Check sheet for the modelled part. Datum: model origin and axes. Units: mm. Face numbers are marked on the shaded views. Give positions to 0.01 mm unless a question says otherwise; leave off trailing zeros. Loops run counter-clockwise (first coordinate to the right, second up) from the corner with the lowest first, then second, coordinate; pieces in that order, holes last. Notation, with made-up numbers: M 18.25,-20.75 L 54.25,-20.75 A32 ccw 54.25,11.25 Z; hole C 72.25,-34.75 d3. An arc over 180 degrees is marked long. Use one line per item in the form item = value.
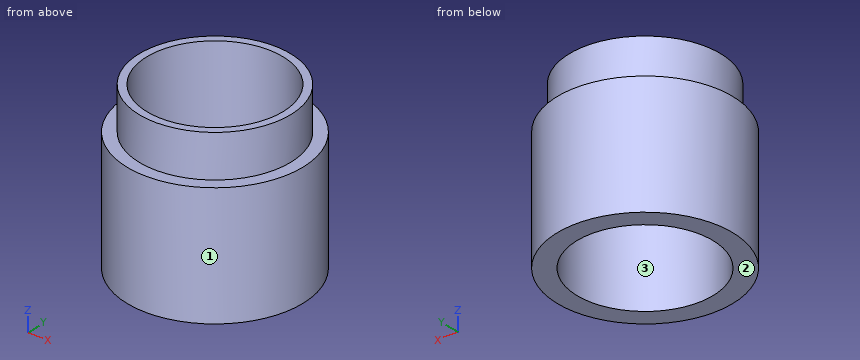
from build123d import *

# Parameters (mm, degrees)
SKETCH1_R           = 14.5
BOSS_EXTRUDE1_DEPTH = 13.5
SKETCH2_OUTSIDE_W   = 40.82
SKETCH2_OUTSIDE_H   = 40.82
SKETCH2_OUTSIDE_R   = 12.5
CUT_EXTRUDE1_DEPTH  = 7
SKETCH3_R           = 11.25
CUT_EXTRUDE2_DEPTH  = 34.904277016


with BuildPart() as part:
    # Sketch1 → Boss-Extrude1 (new, symmetric)
    with BuildSketch(Plane.XY):
        Circle(SKETCH1_R)
    extrude(amount=BOSS_EXTRUDE1_DEPTH, both=True)

    # Sketch2 outside → Cut-Extrude1 (cut)
    with BuildSketch(Plane.XY.offset(13.5)):
        Rectangle(SKETCH2_OUTSIDE_W, SKETCH2_OUTSIDE_H)
        Circle(SKETCH2_OUTSIDE_R, mode=Mode.SUBTRACT)
    extrude(amount=-CUT_EXTRUDE1_DEPTH, mode=Mode.SUBTRACT)

    # Sketch3 → Cut-Extrude2 (cut, through all)
    with BuildSketch(Plane.XY.offset(13.5)):
        Circle(SKETCH3_R)
    extrude(amount=-CUT_EXTRUDE2_DEPTH, mode=Mode.SUBTRACT)


solid = part.part
1) Scan lines: line 1 (Y direction, x = 0, z = 1); line 2 (Y direction, x = 0, z = 7); line 3 (Z direction, x = 7.25, y = 11). Record each from-to range of solid material in increasing order.
Evaluation:
line_1 = -14.5 to -11.25, 11.25 to 14.5
line_2 = -12.5 to -11.25, 11.25 to 12.5
line_3 = -13.5 to 6.5
2) Section check A-A (x = 0). Record the cut outline in (y, z).
Evaluation:
outline = M -14.5,-13.5 L -11.25,-13.5 L -11.25,13.5 L -12.5,13.5 L -12.5,6.5 L -14.5,6.5 Z; M 11.25,-13.5 L 14.5,-13.5 L 14.5,6.5 L 12.5,6.5 L 12.5,13.5 L 11.25,13.5 Z
3) Depth check by flat-ended pin: pin 1 Ø6 at (y, z) = (8.5, -2) entering from -X; pin 2 Ø12 at (x, z) = (2, -2) entering from +Y; pin 3 Ø2 at (x, z) = (8, -3.5) entering from -Y; pin 4 Ø6 at (y, z) = (5, -8) entering from +X. Enter the tip coordinate at first touch or a pass-through.
Evaluation:
pin_1 = -13.42
pin_2 = 14.5
pin_3 = -12.7
pin_4 = 14.36
4) Release check for a two-part mould opening along Y. For the marked faces 1, 2 and 3 record: pulls with the +Y half, pulls with the -Y half, needs draft (parallel to the pull), parting line crosses it, or undercut.
Evaluation:
face_1 = parting line crosses it
face_2 = needs draft
face_3 = undercut
5) Section check C-C (z = -6). Record the cut outline in (x, y), then the cut area to 3 significant figures.
Evaluation:
outline = C 0,0 d29; hole C 0,0 d22.5
area = 263 mm^2
6) Section check D-D (y = -11.75). Record the cut outline in (x, z), then the cut area to 3 significant figures.
Evaluation:
outline = M -8.5,-13.5 L 8.5,-13.5 L 8.5,6.5 L 4.26,6.5 L 4.26,13.5 L -4.26,13.5 L -4.26,6.5 L -8.5,6.5 Z
area = 400 mm^2
